For this review, use the dimensioned drawing (mm, ordinates from the lowest corner) and the shaded views. A direction names the side the tool comes from. Give positions to 0.01 mm unless a question says otherwise; leave off trailing zeros. Order: outer loops, then holes, each group sorted by start corner. A loop starts at its lowest first (then second) coordinate and runs counter-clockwise, first axis right, second up. Notation, with made-up numbers: (16.25, 47) -> (40.25, 47) arc R27 cw to (40.25, 82) -> close; hole circle Ø2 at (80, 21.25). An arc over 180 degrees is marked (long way). Answer as a JSON object with one key per item and string values. Group by question number.
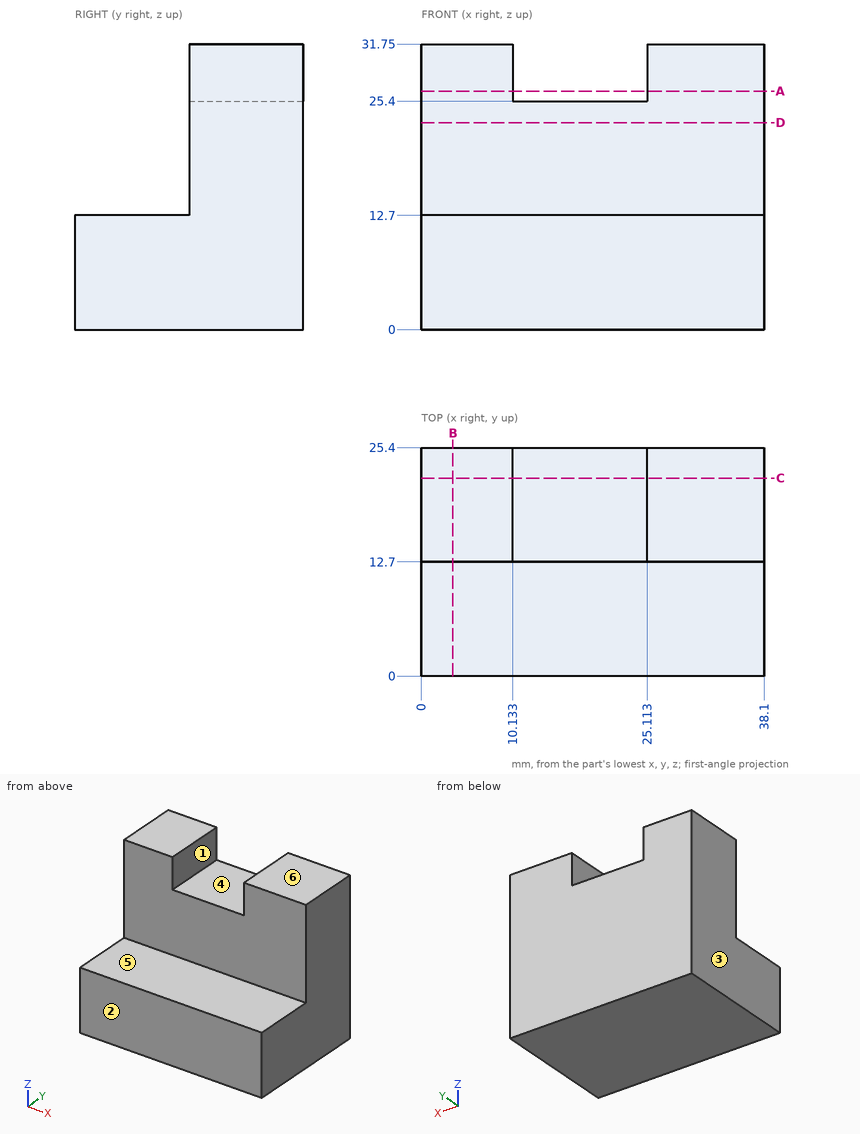
1. Take a section at A-A on z = 26.5. Give the boundary of the cut face in (x, y), plus the area to 3 significant figures.
2. For probe 1 along Z at (x, y) = (25, 5.75); probe 2 along Y at (x, z) = (7.5, 17); probe 3 along X at (y, z) = (22.5, 27.5), list the stretches that pass through material, from the lowest coordinate up. Write a range as [from, to].
3. For pin 1 (6.5 mm diameter, centred on x = 14, y = 21, fed in from +Z); pin 2 (4 mm diameter, centred on x = 9.5, y = 8.5, fed in from +Z); pin 3 (9.5 mm diameter, centred on x = 16.5, z = 24.5, fed in from -Y), all flat-tipped, find the tip position at first contact; note any pin that passes through.
4. Take a section at D-D on z = 23. Give the boundary of the cut face in (x, y), plus the area to 3 significant figures.
5. Machinability: for the marked faces 4, 5 and 6, which of the approach directions +Z, -Z, +X, -X, +Y, -Y give a long, thin tool a straight path to every point of the face, cutting with its end or side? Answer none if there is none.
6. Take a section at C-C on y = 22. Give the boundary of the cut face in (x, z), plus the area to 3 significant figures.
7. Take a section at B-B on x = 3.5. Give the boundary of the cut face in (y, z).
8. Draft analysis for pull direction X (two halves, no side actions). For the marked faces 1, 2 and 3, state which applies: pulls with the +X half, pulls with the -X half, needs draft (parallel to the pull), parting line crosses it, or undercut.
Checks:
{
 "1": {"outline": "(0, 12.7) -> (10.13, 12.7) -> (10.13, 25.4) -> (0, 25.4) -> close; (25.11, 12.7) -> (38.1, 12.7) -> (38.1, 25.4) -> (25.11, 25.4) -> close", "area": "294 mm2"},
 "2": {"probe 1": "z = [0, 12.7]", "probe 2": "y = [12.7, 25.4]", "probe 3": "x = [0, 10.13], [25.11, 38.1]"},
 "3": {"pin 1": "stops at z = 25.4", "pin 2": "stops at z = 12.7", "pin 3": "stops at y = 12.7"},
 "4": {"outline": "(0, 12.7) -> (38.1, 12.7) -> (38.1, 25.4) -> (0, 25.4) -> close", "area": "484 mm2"},
 "5": {"face 4": "+Z, +Y, -Y", "face 5": "+Z, +X, -X, -Y", "face 6": "+Z, +X, -X, +Y, -Y"},
 "6": {"outline": "(0, 0) -> (38.1, 0) -> (38.1, 31.75) -> (25.11, 31.75) -> (25.11, 25.4) -> (10.13, 25.4) -> (10.13, 31.75) -> (0, 31.75) -> close", "area": "1,110 mm2"},
 "7": {"outline": "(0, 0) -> (25.4, 0) -> (25.4, 31.75) -> (12.7, 31.75) -> (12.7, 12.7) -> (0, 12.7) -> close"},
 "8": {"face 1": "undercut", "face 2": "needs draft", "face 3": "pulls with the -X half"}
}
